Geometry check sheet. Reference: drawing and pictorial views, mm from the part's lowest x, y, z. A direction names the side the tool comes from. Coordinates: 2 decimals unless noted, no trailing zeros. Loops run counter-clockwise (first coordinate to the right, second up) from the corner with the lowest first, then second, coordinate; pieces in that order, holes last. Notation, with made-up numbers: (13.25, -4) -> (51.25, -4) arc R17 cw to (51.25, 26) -> close; hole circle Ø8 at (52, 71.25). An arc over 180 degrees is marked (long way). Answer as a JSON object with one key per item and string values.
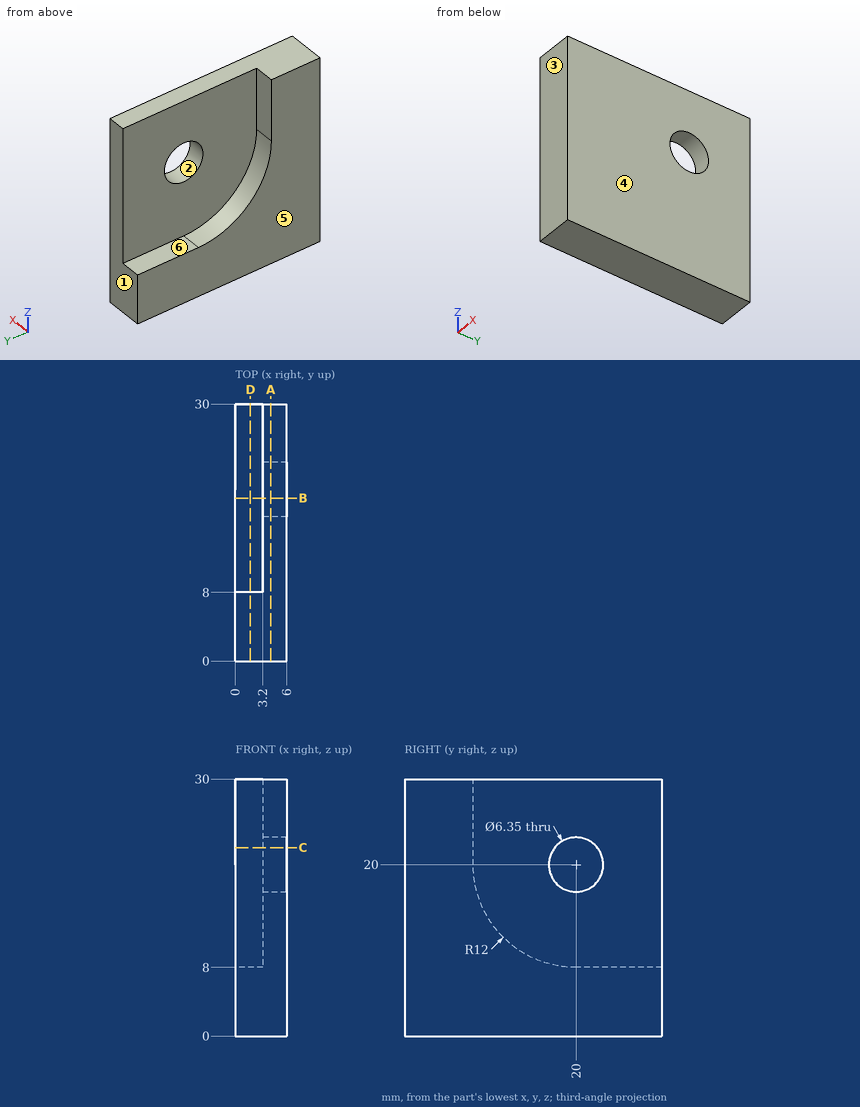
1. Depth check by flat-ended pin: P1, Ø3.5, axis at x = 1, y = 24, coming from the +Z side; P2, Ø1.5, axis at x = 2, y = 17, coming from the +Z side; P3, Ø3, axis at y = 11, z = 20.5, coming from the -X side. Enter the tip coordinate at first touch or a pass-through.
Evaluation:
{"P1": "stops at z = 8", "P2": "stops at z = 8.6", "P3": "stops at x = 3.2"}
2. Tool access check on the marked faces 5 and 6. Record the directions out of +Z, -Z, +X, -X, +Y, -Y that give a thin tool (end or side, any length) a straight path to the whole face; none if there is none.
Evaluation:
{"face 5": "+Z, -Z, -X, +Y, -Y", "face 6": "+Z, -X, +Y"}
3. Section check A-A, the plane x = 4.15. Record the boundary of the cut face in (y, z) (3 decimals), then the cut area to 3 significant figures.
Evaluation:
{"outline": "(0, 0) -> (30, 0) -> (30, 30) -> (0, 30) -> close; hole circle Ø6.35 at (20, 20)", "area": "868 mm^2"}
4. Section check B-B, the plane y = 19. Record the boundary of the cut face in (x, z).
Evaluation:
{"outline": "(0, 0) -> (6, 0) -> (6, 16.99) -> (3.2, 16.99) -> (3.2, 8.04) -> (0, 8.04) -> close; (3.2, 23.01) -> (6, 23.01) -> (6, 30) -> (3.2, 30) -> close"}
5. Thickness scan on probe 1 along Y at (x, z) = (4.15, 20) (3 decimals); probe 2 along X at (y, z) = (18.75, 14); probe 3 along Z at (x, y) = (3.55, 18.75). Record the ranges inside material, lowest first. Write a range as from..to.
Evaluation:
{"probe 1": "y = 0..16.825, 23.175..30", "probe 2": "x = 3.2..6", "probe 3": "z = 0..17.08, 22.92..30"}
6. Section check C-C, the plane z = 22. Record the boundary of the cut face in (x, y), then the cut area to 3 significant figures.
Evaluation:
{"outline": "(0, 0) -> (6, 0) -> (6, 17.53) -> (3.2, 17.53) -> (3.2, 8) -> (0, 8) -> close; (3.2, 22.47) -> (6, 22.47) -> (6, 30) -> (3.2, 30) -> close", "area": "95.8 mm^2"}
7. Mould release check, pull along Y, two halves, no side actions. Record for the marked faces 1, 2, 3 and 4: released by +Y, released by -Y, zero draft, split by the parting line, or undercut.
Evaluation:
{"face 1": "released by +Y", "face 2": "undercut", "face 3": "released by -Y", "face 4": "zero draft"}
8. Section check D-D, the plane x = 1.75. Record the boundary of the cut face in (y, z).
Evaluation:
{"outline": "(0, 0) -> (30, 0) -> (30, 8) -> (20, 8) arc R12 cw to (8, 20) -> (8, 30) -> (0, 30) -> close"}
